The listing builds one solid part. Answer for the finished solid, in the listing's coordinates (mm). A direction names the side the tool comes from. Coordinates: 2 decimals unless noted, no trailing zeros. Write each loop counter-clockwise with the first axis right and the second up, starting at its lowest first coordinate (ties: lowest second). Pieces come first, ordered by that corner, then holes.
```python
from build123d import *

# Parameters (mm, degrees)
F0_W     = 18
F0_H     = 9
F0_R     = 1.75
F1_DEPTH = 5
F2_R     = 1.75
F3_DEPTH = 1.5
F4_SIZE  = 1


with BuildPart() as f1:
    # F0 (on Top) → F1 (new body)
    with BuildSketch(Plane.XY):
        Rectangle(F0_W, F0_H)
        with Locations((-6, 0)):
            Circle(F0_R, mode=Mode.SUBTRACT)
        with Locations((6, 0)):
            Circle(F0_R, mode=Mode.SUBTRACT)
    extrude(amount=F1_DEPTH)

    # F2 (on face) → F3 (cut)
    with BuildSketch(Plane.XY.offset(5)):
        Polygon((-8.9, 1.674316), (-8.9, -1.674316), (-6, -3.348632), (-3.1, -1.674316), (-3.1, 1.674316), (-6, 3.348632), align=None)
        with Locations((-6, 0)):
            Circle(F2_R, mode=Mode.SUBTRACT)
        Polygon((3.1, 1.674316), (3.1, -1.674316), (6, -3.348632), (8.9, -1.674316), (8.9, 1.674316), (6, 3.348632), align=None)
        with Locations((6, 0)):
            Circle(F2_R, mode=Mode.SUBTRACT)
    extrude(amount=-F3_DEPTH, mode=Mode.SUBTRACT)

    # F4
    f4_edges = [f1.edges().sort_by_distance(p)[0] for p in [
        (0, -4.5, 0),
        (0, 4.5, 0),
    ]]
    chamfer(f4_edges, length=F4_SIZE)


solid = f1.part
```
(1) For a pull along X with two mould halves and no side action, classify faces 1 (the flat face through (9, 0, 2)), 2 (the flat face through (0, 0, 5)), 3 (the flat face through (-4.57, -2.523, 4.26)) as pulls with the +X half, pulls with the -X half, needs draft (parallel to the pull), parting line crosses it, or undercut.
(2) Section B-B, the plane z = 4.3 is taken. Write down the section's boundary in (x, y).
(3) Section C-C, the plane x = 2.25 is taken. Write down the section's boundary in (y, z), plus the area to 3 significant figures.
(4) Find the intervals of material crossed by probe 1 along Y at (x, z) = (6, 2.15); probe 2 along Z at (x, y) = (7.5, -1); probe 3 along Y at (x, z) = (4.5, 0.7), in increasing order.
(5) Section A-A, the plane y = 0 is taken. Write down the section's boundary in (x, z).
(6) Each of these flat-tipped pins is pushed along its axis until it touches: pin 1 (1.7 mm diameter, centred on x = -6, y = -0.5, fed in from +Z); pin 2 (3 mm diameter, centred on x = 5, y = 0.5, fed in from +Z); pin 3 (2 mm diameter, centred on x = -6.5, y = -3, fed in from +Z). Where does it stop, or does it pass through?
(7) Which of the six approach directions +Z, -Z, +X, -X, +Y, -Y give full straight-line access (tool end or side, diameter ignored) to faces 4 (the flat face through (7.43, -2.523, 4.26)), 5 (the flat face through (-0.1, 4, 0.5))?
(8) Section D-D, the plane x = -7 is taken. Write down the section's boundary in (y, z).
Solution:
1. face 1: pulls with the +X half
1. face 2: needs draft
1. face 3: undercut
2. outline: (-9, -4.5) - (9, -4.5) - (9, 4.5) - (-9, 4.5) - close; hole (-8.9, -1.67) - (-6, -3.35) - (-3.1, -1.67) - (-3.1, 1.67) - (-6, 3.35) - (-8.9, 1.67) - close; hole (3.1, -1.67) - (6, -3.35) - (8.9, -1.67) - (8.9, 1.67) - (6, 3.35) - (3.1, 1.67) - close
3. outline: (-4.5, 1) - (-3.5, 0) - (3.5, 0) - (4.5, 1) - (4.5, 5) - (-4.5, 5) - close
3. area: 44.0 mm2
4. probe 1: y = -4.5 to -1.75, 1.75 to 4.5
4. probe 2: z = 0 to 3.5
4. probe 3: y = -4.2 to -0.9, 0.9 to 4.2
5. outline: (-9, 0) - (-7.75, 0) - (-7.75, 3.5) - (-8.9, 3.5) - (-8.9, 5) - (-9, 5) - close; (-4.25, 0) - (4.25, 0) - (4.25, 3.5) - (3.1, 3.5) - (3.1, 5) - (-3.1, 5) - (-3.1, 3.5) - (-4.25, 3.5) - close; (7.75, 0) - (9, 0) - (9, 5) - (8.9, 5) - (8.9, 3.5) - (7.75, 3.5) - close
6. pin 1: passes through
6. pin 2: stops at z = 3.5
6. pin 3: stops at z = 5
7. face 4: +Z
7. face 5: -Z, +X, -X, +Y
8. outline: (-4.5, 1) - (-3.5, 0) - (-1.44, 0) - (-1.44, 3.5) - (-2.77, 3.5) - (-2.77, 5) - (-4.5, 5) - close; (1.44, 0) - (3.5, 0) - (4.5, 1) - (4.5, 5) - (2.77, 5) - (2.77, 3.5) - (1.44, 3.5) - close
